Design review of the part built by this model. Coordinates are the model's own, in mm. A direction names the side the tool comes from. Coordinates: 2 decimals unless noted, no trailing zeros. Order: outer loops, then holes, each group sorted by start corner. A loop starts at its lowest first (then second) coordinate and runs counter-clockwise, first axis right, second up. Notation, with made-up numbers: M 55,-21 L 87,-21 A24 cw 87,-2 Z; hole C -7,-36.75 d2. An arc over 180 degrees is marked long. Use CSV: the item, a comma, the result in double quotes.
```python
from build123d import *

# Parameters (mm, degrees)
F1_DEPTH    = 38.1
F2_T1_DEPTH = 38.1
F2_T3_DEPTH = 50.8
F3_T1_DEPTH = 38.1
F4_R        = 1.26999
F5_W        = 23.6700927116
F5_H        = 11.2887102096
F6_DEPTH    = 38.101
F7_R        = 2.54


# Not quite as in the source:
# - a fillet or chamfer that OpenCascade refuses, or shapes differently, is made with other operations: its cross-section is extruded or revolved along the edge and cut away or added
# - a fillet or chamfer is up to 0.001 mm smaller than in the source, because OpenCascade refuses the exact size


with BuildPart() as f1:
    # F0 (on Top) → F1 (new body)
    with BuildSketch(Plane.XY):
        Polygon((-36.3474, 25.4), (-36.3474, 0), (36.3474, 0), (36.3474, 12.7), (32.5374, 13.3656184486), (32.5374, 2.54), (29.337, 2.54), (29.337, 13.9247379455), (26.797, 14.3684835779), (26.797, 2.54), (23.0886, 2.54), (23.0886, 15.0163522013), (19.2786, 15.6819706499), (19.2786, 2.54), (14.7066, 2.54), (14.7066, 16.4807127883), (12.1666, 16.9244584207), (12.1666, 2.54), (7.5946, 2.54), (7.5946, 17.723200559), (5.0546, 18.1669461915), (5.0546, 2.54), (0.4826, 2.54), (0.4826, 18.9656883298), (-2.0574, 19.4094339623), (-2.0574, 2.54), (-7.1374, 2.54), (-7.1374, 20.2969252271), (-9.6774, 20.7406708595), (-9.6774, 2.54), (-14.7574, 2.54), (-14.7574, 21.6281621244), (-17.2974, 22.0719077568), (-17.2974, 2.54), (-23.6474, 2.54), (-23.6474, 23.1812718379), (-26.1874, 23.6250174703), (-26.1874, 2.54), (-32.5374, 2.54), (-32.5374, 24.9766666667), align=None)
    extrude(amount=F1_DEPTH)

    # F2: fillet of radius 2.54 on 14 edges, made by hand

    # F2_s2 → F2_t1 (join)
    with BuildSketch(Plane.XY):
        with BuildLine():
            ThreePointArc((-29.9974, 2.54), (-31.7934512242, 3.2839487758), (-32.5374, 5.08))
            Line((-32.5374, 5.08), (-32.5374, 2.54))
            Line((-32.5374, 2.54), (-29.9974, 2.54))
        make_face()
        with BuildLine():
            ThreePointArc((-26.1874, 5.08), (-26.9313487758, 3.2839487758), (-28.7274, 2.54))
            Line((-28.7274, 2.54), (-26.1874, 2.54))
            Line((-26.1874, 2.54), (-26.1874, 5.08))
        make_face()
        with BuildLine():
            ThreePointArc((-21.1074, 2.54), (-22.9034512242, 3.2839487758), (-23.6474, 5.08))
            Line((-23.6474, 5.08), (-23.6474, 2.54))
            Line((-23.6474, 2.54), (-21.1074, 2.54))
        make_face()
        with BuildLine():
            ThreePointArc((-17.2974, 5.08), (-18.0413487758, 3.2839487758), (-19.8374, 2.54))
            Line((-19.8374, 2.54), (-17.2974, 2.54))
            Line((-17.2974, 2.54), (-17.2974, 5.08))
        make_face()
        with BuildLine():
            ThreePointArc((-12.2174, 2.54), (-14.0134512242, 3.2839487758), (-14.7574, 5.08))
            Line((-14.7574, 5.08), (-14.7574, 2.54))
            Line((-14.7574, 2.54), (-12.2174, 2.54))
        make_face()
        with BuildLine():
            ThreePointArc((-9.6774, 5.08), (-10.4213487758, 3.2839487758), (-12.2174, 2.54))
            Line((-12.2174, 2.54), (-9.6774, 2.54))
            Line((-9.6774, 2.54), (-9.6774, 5.08))
        make_face()
        with BuildLine():
            ThreePointArc((-4.5974, 2.54), (-6.3934512242, 3.2839487758), (-7.1374, 5.08))
            Line((-7.1374, 5.08), (-7.1374, 2.54))
            Line((-7.1374, 2.54), (-4.5974, 2.54))
        make_face()
        with BuildLine():
            ThreePointArc((-2.0574, 5.08), (-2.8013487758, 3.2839487758), (-4.5974, 2.54))
            Line((-4.5974, 2.54), (-2.0574, 2.54))
            Line((-2.0574, 2.54), (-2.0574, 5.08))
        make_face()
        with BuildLine():
            ThreePointArc((3.0226, 2.54), (1.2265487758, 3.2839487758), (0.4826, 5.08))
            Line((0.4826, 5.08), (0.4826, 2.54))
            Line((0.4826, 2.54), (3.0226, 2.54))
        make_face()
        with BuildLine():
            ThreePointArc((5.0546, 5.08), (4.3106512242, 3.2839487758), (2.5146, 2.54))
            Line((2.5146, 2.54), (5.0546, 2.54))
            Line((5.0546, 2.54), (5.0546, 5.08))
        make_face()
        with BuildLine():
            ThreePointArc((10.1346, 2.54), (8.3385487758, 3.2839487758), (7.5946, 5.08))
            Line((7.5946, 5.08), (7.5946, 2.54))
            Line((7.5946, 2.54), (10.1346, 2.54))
        make_face()
        with BuildLine():
            ThreePointArc((12.1666, 5.08), (11.4226512242, 3.2839487758), (9.6266, 2.54))
            Line((9.6266, 2.54), (12.1666, 2.54))
            Line((12.1666, 2.54), (12.1666, 5.08))
        make_face()
    extrude(amount=F2_T1_DEPTH)

    # F2_s4 → F2_t3 (cut)
    with BuildSketch(Plane.XY.offset(-6.35)):
        with BuildLine():
            ThreePointArc((-33.8074, 0), (-35.6034512242, 0.7439487758), (-36.3474, 2.54))
            Line((-36.3474, 2.54), (-36.3474, 0))
            Line((-36.3474, 0), (-33.8074, 0))
        make_face()
        with BuildLine():
            ThreePointArc((36.3474, 2.54), (35.6034512242, 0.7439487758), (33.8074, 0))
            Line((33.8074, 0), (36.3474, 0))
            Line((36.3474, 0), (36.3474, 2.54))
        make_face()
    extrude(amount=F2_T3_DEPTH, mode=Mode.SUBTRACT)

    # F3: fillet of radius 1.778 on 6 edges, made by hand

    # F3_s2 → F3_t1 (join)
    with BuildSketch(Plane.XY):
        with BuildLine():
            ThreePointArc((14.7066, 4.318), (15.2273641431, 3.0607641431), (16.4846, 2.54))
            Line((16.4846, 2.54), (14.7066, 2.54))
            Line((14.7066, 2.54), (14.7066, 4.318))
        make_face()
        with BuildLine():
            ThreePointArc((17.5006, 2.54), (18.7578358569, 3.0607641431), (19.2786, 4.318))
            Line((19.2786, 4.318), (19.2786, 2.54))
            Line((19.2786, 2.54), (17.5006, 2.54))
        make_face()
        with BuildLine():
            ThreePointArc((23.0886, 4.318), (23.6093641431, 3.0607641431), (24.8666, 2.54))
            Line((24.8666, 2.54), (23.0886, 2.54))
            Line((23.0886, 2.54), (23.0886, 4.318))
        make_face()
        with BuildLine():
            ThreePointArc((25.019, 2.54), (26.2762358569, 3.0607641431), (26.797, 4.318))
            Line((26.797, 4.318), (26.797, 2.54))
            Line((26.797, 2.54), (25.019, 2.54))
        make_face()
        with BuildLine():
            ThreePointArc((29.337, 4.318), (29.8577641431, 3.0607641431), (31.115, 2.54))
            Line((31.115, 2.54), (29.337, 2.54))
            Line((29.337, 2.54), (29.337, 4.318))
        make_face()
        with BuildLine():
            ThreePointArc((30.7594, 2.54), (32.0166358569, 3.0607641431), (32.5374, 4.318))
            Line((32.5374, 4.318), (32.5374, 2.54))
            Line((32.5374, 2.54), (30.7594, 2.54))
        make_face()
    extrude(amount=F3_T1_DEPTH)

    # F4 (radius 1.27 in the source; OpenCascade refuses exactly that, so slightly less here)
    f4_edges = [f1.edges().sort_by_distance(p)[0] for p in [
        (32.5374, 13.365618, 19.05),
        (29.337, 13.924738, 19.05),
        (26.797, 14.368484, 19.05),
        (23.0886, 15.016352, 19.05),
        (19.2786, 15.681971, 19.05),
        (14.7066, 16.480713, 19.05),
        (12.1666, 16.924458, 19.05),
        (7.5946, 17.723201, 19.05),
        (5.0546, 18.166946, 19.05),
        (0.4826, 18.965688, 19.05),
        (-2.0574, 19.409434, 19.05),
        (-7.1374, 20.296925, 19.05),
        (-14.7574, 21.628162, 19.05),
        (-23.6474, 23.181272, 19.05),
        (-26.1874, 23.625017, 19.05),
        (-32.5374, 24.976667, 19.05),
        (-36.3474, 25.4, 19.05),
        (36.3474, 12.7, 19.05),
        (-9.6774, 20.740671, 19.05),
        (-17.2974, 22.071908, 19.05),
    ]]
    fillet(f4_edges, radius=F4_R)

    # F5 (on face) → F6 (cut, through all)
    with BuildSketch(Plane.XY.offset(38.1)):
        with Locations((34.9236463558, 19.5933448658)):
            Rectangle(F5_W, F5_H)
        Polygon((46.7586927116, 13.948989761), (23.0886, 13.948989761), (23.0886, -14.5505452529), (53.0812069774, -14.5505452529), (53.0812069774, 13.948989761), align=None)
    extrude(amount=-F6_DEPTH, mode=Mode.SUBTRACT)

    # F7
    f7_edges = [f1.edges().sort_by_distance(p)[0] for p in [
        (23.0886, 0, 19.05),
    ]]
    fillet(f7_edges, radius=F7_R)


solid = f1.part
```
(1) Add section C-C on x = -3. State the section outline as (y, z) points.
The answers:
outline,"M 0,0 L 3.11,0 L 3.11,38.1 L 0,38.1 Z"
(2) Add section A-A on y = 12.75. Give the number of separate pieces and of enclosed holes in the cut face, and give its area (3 significant figures).
The answers:
separate pieces,"8"
enclosed holes,"0"
area,"871 mm2"
(3) The part is to be moulded in two halves that separate along X. For faces 3 (the face through (22.78, 14.78, 19.32)), 4 (the face through (19.279, 9, 19)), say which applies: pulls with the +X half, pulls with the -X half, needs draft (parallel to the pull), parting line crosses it, or undercut.
The answers:
face 3,"pulls with the +X half"
face 4,"undercut"
(4) Clearance check with flat-ended pins moving along their axes: P1, Ø5, axis at y = 17, z = 18, coming from the +X side; P2, Ø1.1, axis at x = 17, z = 24, coming from the +Y side; P3, Ø1, axis at x = -14.5, z = 28, coming from the +Y side. State where each tip first meets the part, or that it passes through.
The answers:
P1,"stops at x = 22.96"
P2,"stops at y = 2.54"
P3,"stops at y = 21.31"
(5) Wall thickness on probe 1 along X at (y, z) = (17.25, 22); probe 2 along X at (y, z) = (17, 28); probe 3 along X at (y, z) = (18.5, 5.5): over which ranges is each line inside the solid? List them lowest first.
The answers:
probe 1,"x = -36.35 to -32.54, -26.19 to -23.65, -17.3 to -14.76, -9.68 to -7.14, -2.06 to 0.48, 5.2 to 7.45"
probe 2,"x = -36.35 to -32.54, -26.19 to -23.65, -17.3 to -14.76, -9.68 to -7.14, -2.06 to 0.48, 5.1 to 7.55"
probe 3,"x = -36.35 to -32.54, -26.19 to -23.65, -17.3 to -14.76, -9.68 to -7.14, -1.91 to 0.33"
(6) Add section B-B on x = -18.5. State the section outline as (y, z) points, and give its area (3 significant figures).
The answers:
outline,"M 0,0 L 2.92,0 L 2.92,38.1 L 0,38.1 Z"
area,"111 mm2"
(7) For faces 1 (the face through (-32.537, 14, 19)), 2 (the face through (-7.443, 20.056, 19.317)), list the 3-axis set-ups (+Z, -Z, +X, -X, +Y, -Y) from which the entire face can be reached by the end or side of a thin tool; tool diameter is ignored.
The answers:
face 1,"+Z, -Z, +Y"
face 2,"+Z, -Z, +X, +Y"
